Source: CAD feature listing. Evaluate the final solid. Frame: model axes, mm. A direction names the side the tool comes from. Coordinates: 2 decimals unless noted, no trailing zeros. Write each loop counter-clockwise with the first axis right and the second up, starting at its lowest first coordinate (ties: lowest second). Pieces come first, ordered by that corner, then holes. Notation, with made-up numbers: M -4.5,-19 L 29.5,-19 A28 ccw 29.5,13 Z; hole C 77.25,16.5 d1. An arc over 180 degrees is marked long. One line per item, written item: value. Start each with the question number.
Item 1: Pin query (flat end, axial travel): P1, Ø1.5, axis at x = -1.5, y = -1.5, coming from the -Z side; P2, Ø0.9, axis at x = 1, z = 3, coming from the -Y side; P3, Ø1, axis at x = -1, y = -1.5, coming from the -Z side; P4, Ø3, axis at y = -4, z = 2.5, coming from the -X side. Return the tip coordinate at first contact, or that it passes through.
Item 2: Cut plane B-B, the plane x = 0. Output: boundary loops of the cut face in (y, z) (3 decimals), then the cut area to 3 significant figures.
Item 3: Cut plane A-A, the plane z = 5. Output: boundary loops of the cut face in (x, y) (3 decimals), then the cut area to 3 significant figures.
Item 4: Cut plane D-D, the plane z = 7.75. Output: boundary loops of the cut face in (x, y) (3 decimals).
Item 5: Cut plane C-C, the plane y = -1. Output: boundary loops of the cut face in (x, z) (3 decimals).
Item 6: Ray query, L1, parallel to Y at x = 0, z = 4; L2, parallel to Y at x = 0, z = 9.5 (3 decimals); L3, parallel to Z at x = -0.75, y = 1.25. Return the intervals inside material, ascending. Write a range as from..to.
Item 7: Set-up query: faces 1 (the flat face through (0, -1, 14)), 2 (the cylindrical face through (0.1, -2.6, 6.1)). Return all of +Z, -Z, +X, -X, +Y, -Y with unobstructed straight access to the full face (end or side cutting, diameter ignored); none if empty.
Item 8: Mould query, pull axis Y, two halves, no side actions, for faces 3 (the flat face through (0, 0, 12)), 4 (the flat face through (0, 3, 0)). Classes: released by +Y, released by -Y, zero draft, split by the parting line, or undercut.
```python
from build123d import *

# Parameters (mm, degrees)
ESQUISSE1_R             = 3.975
BOSS_EXTRU_1_DEPTH      = 7
ESQUISSE2_R             = 3.975
BOSS_EXTRU_2_DEPTH      = 7
ENL_V_START             = -2
ENL_V_MAT_EXTRU_1_DEPTH = 14.38022269
CHANFREIN2_SIZE         = 1.75
CHANFREIN4_SIZE         = 1.75


with BuildPart() as part:
    # Esquisse1 → Boss.-Extru.1 (new body)
    with BuildSketch(Plane.XY):
        with Locations((0, 0.822072072)):
            Circle(ESQUISSE1_R)
    extrude(amount=BOSS_EXTRU_1_DEPTH)

    # Esquisse2 → Boss.-Extru.2 (add)
    with BuildSketch(Plane.XY.offset(7)):
        with Locations(Location((0, -1, 0), (0, 0, 166.750525957))):
            Circle(ESQUISSE2_R)
    extrude(amount=BOSS_EXTRU_2_DEPTH)

    # Esquisse3 → Enlèv. mat.-Extru.1 (cut, through all)
    with BuildSketch(Plane.XY.offset(14).offset(ENL_V_START)):
        with BuildLine():
            Line((-1.532970972, 2.1), (1.532970972, 2.1))
            ThreePointArc((1.532970972, 2.1), (0, -2.6), (-1.532970972, 2.1))
        make_face()
    extrude(amount=-ENL_V_MAT_EXTRU_1_DEPTH, mode=Mode.SUBTRACT)

    # Chanfrein2
    # the kernel refuses this chamfer: 1.75 mm, written as the material it takes off along each edge
    with BuildSketch(Plane(origin=(0, 0.822072072, 7), x_dir=(1, 0, 0), z_dir=(0, -1, 0))) as chanfrein2_piece_1_section:
        Polygon((3.975, -CHANFREIN2_SIZE), (3.975 - CHANFREIN2_SIZE, 0), (3.975, 0), align=None)
    chanfrein2_piece_1 = revolve(axis=Axis((0, 0.822072072, 7), (0, 0, 1)), revolution_arc=258.239304613, mode=Mode.PRIVATE)
    chanfrein2_piece_1 = chanfrein2_piece_1 - Plane(origin=(0, -1, 6.142541617), x_dir=(-0.9733813624059963, 0.22919145560130838, 0), z_dir=(0, 0, -1)) * Cylinder(3.975, 16, mode=Mode.PRIVATE)
    add(chanfrein2_piece_1, mode=Mode.SUBTRACT)
    with BuildSketch(Plane(origin=(0, 0.822072072, 7), x_dir=(0.20586939253859726, -0.9785794772095873, 0), z_dir=(-0.9785794772095873, -0.20586939253859726, 0))) as chanfrein2_piece_2_section:
        Polygon((3.975, -CHANFREIN2_SIZE), (3.975 - CHANFREIN2_SIZE, 0), (3.975, 0), align=None)
    chanfrein2_piece_2 = revolve(axis=Axis((0, 0.822072072, 7), (0, 0, 1)), revolution_arc=78.119602811, mode=Mode.PRIVATE)
    chanfrein2_piece_2 = chanfrein2_piece_2 - Plane(origin=(0, -1, 6.194476716), x_dir=(-0.9733813624059963, 0.22919145560130838, 0), z_dir=(0, 0, -1)) * Cylinder(3.975, 16, mode=Mode.PRIVATE)
    add(chanfrein2_piece_2, mode=Mode.SUBTRACT)

    # Chanfrein4
    # the kernel refuses this chamfer: 1.75 mm, written as the material it takes off along each edge
    with BuildSketch(Plane(origin=(0, -1, 7), x_dir=(-0.2035326199648153, 0.9790681654564498, 0), z_dir=(0.9790681654564498, 0.2035326199648153, 0))) as chanfrein4_piece_1_section:
        Polygon((3.975 - CHANFREIN4_SIZE, 0), (3.975, CHANFREIN4_SIZE), (3.975, 0), align=None)
    chanfrein4_piece_1 = revolve(axis=Axis((0, -1, 7), (0, 0, 1)), revolution_arc=336.512773019, mode=Mode.PRIVATE)
    chanfrein4_piece_1 = chanfrein4_piece_1 - Plane(origin=(0, 0.822072072, 7.857337324), x_dir=(1, 0, 0), z_dir=(0, 0, -1)) * Cylinder(3.975, 16, mode=Mode.PRIVATE)
    add(chanfrein4_piece_1, mode=Mode.SUBTRACT)


solid = part.part
```
From the geometry:
1. P1: stops at z = 0
1. P2: stops at y = -3.11
1. P3: stops at z = 12
1. P4: stops at x = -2.18
2. outline: M -4.975,8.75 L -3.225,7 L -3.153,7 L -3.153,0 L -2.6,0 L -2.6,12 L 2.1,12 L 2.1,0 L 4.797,0 L 4.797,5.25 L 3.047,7 L 2.975,7 L 2.975,14 L -4.975,14 Z
2. area: 51.8 mm²
3. outline: C 0,0.822 d7.95; hole M -1.533,2.1 A2.6 ccw long 1.533,2.1 Z
3. area: 29.4 mm²
4. outline: M -3.869,-0.089 A3.975 ccw -2.803,-1.996 A2.975 ccw 2.803,-1.996 A3.975 ccw 3.869,-0.089 A3.975 ccw Z; hole M -1.533,2.1 A2.6 ccw long 1.533,2.1 Z
5. outline: M -3.975,8.75 L -3.533,8.308 L -3.533,0 L -2.4,0 L -2.4,12 L 2.4,12 L 2.4,0 L 3.533,0 L 3.533,8.308 L 3.975,8.75 L 3.975,14 L -3.975,14 Z
6. L1: y = -3.15..-2.6, 2.1..4.8
6. L2: y = -4.975..-2.6, 2.1..2.975
6. L3: z = 12..14
7. face 1: +Z, +X, -X, +Y, -Y
7. face 2: -Z
8. face 3: undercut
8. face 4: zero draft
